Model file for the job. Use its own axes, mm. A direction names the side the tool comes from. Round coordinates to 2 decimals unless told otherwise and drop trailing zeros. Order: outer loops, then holes, each group sorted by start corner. A loop starts at its lowest first (then second) coordinate and runs counter-clockwise, first axis right, second up. Notation, with made-up numbers: (-2.75, -5) - (29.25, -5) arc R32 ccw to (29.25, 23) - close; hole circle Ø8 at (72, -37). An arc over 180 degrees is marked (long way). Answer as CSV lines item,"result". Start each with the question number.
1. Pull direction Z, two halves, no side cores. Call faces 1 (the face through (-1, 3, -63.5)), 2 (the face through (-1, 6.35, -1)), 3 (the face through (22.225, 3, -44)): released by +Z, released by -Z, zero draft, split by the parting line, or undercut.
2. 3-axis set-ups, long thin cutter, end or side, ignore diameter. For faces 4 (the face through (-36.141, 3.131, 28.333)), 5 (the face through (22.225, 3, -25)): which of +Z, -Z, +X, -X, +Y, -Y reach the whole face in a straight line?
3. Pin check, flat tips, straight feed: pin 1 Ø5 at (x, z) = (15.875, 0) entering from +Y (3 decimals); pin 2 Ø1.3 at (y, z) = (4, -7.5) entering from +X (3 decimals). Stop position of each tip, or through.
4. Wall check: line 1 along X through (y, z) = (4.5, 0) (3 decimals); line 2 along Z through (x, y) = (29, 5); line 3 along Z through (x, y) = (30, 3.5). Give the ranges that are in metal, low to high. Write a range as [from, to].
5. Band-saw the part on A-A on z = 0. List the corners of the cut face in (x, y) (3 decimals).
6. Band-saw the part on B-B on z = -26. List the corners of the cut face in (x, y) (3 decimals).
```python
from build123d import *

# Parameters (mm, degrees)
SKETCH1_W           = 95.25
SKETCH1_H           = 127
SKETCH1_R           = 3.175
BOSS_EXTRUDE1_DEPTH = 6.35
SKETCH2_R           = 2.15265
CUT_EXTRUDE1_DEPTH  = 25.4


with BuildPart() as part:
    # Sketch1 → Boss-Extrude1 (new body)
    with BuildSketch(Plane(origin=(0, 0, 0), x_dir=(1, 0, 0), z_dir=(0, 1, 0))):
        Rectangle(SKETCH1_W, SKETCH1_H)
        with Locations(Location((-34.925, 0, 0), (0, 0, 270))):
            Circle(SKETCH1_R, mode=Mode.SUBTRACT)
        with Locations(Location((-9.525, 0, 0), (0, 0, 270))):
            Circle(SKETCH1_R, mode=Mode.SUBTRACT)
        with Locations(Location((15.875, 0, 0), (0, 0, 270))):
            Circle(SKETCH1_R, mode=Mode.SUBTRACT)
        with Locations(Location((-9.525, -25.4, 0), (0, 0, 270))):
            Circle(SKETCH1_R, mode=Mode.SUBTRACT)
        with Locations(Location((15.875, -25.4, 0), (0, 0, 270))):
            Circle(SKETCH1_R, mode=Mode.SUBTRACT)
        with Locations(Location((-9.525, -50.8, 0), (0, 0, 270))):
            Circle(SKETCH1_R, mode=Mode.SUBTRACT)
        with Locations(Location((15.875, -50.8, 0), (0, 0, 270))):
            Circle(SKETCH1_R, mode=Mode.SUBTRACT)
        with Locations(Location((-34.925, -25.4, 0), (0, 0, 270))):
            Circle(SKETCH1_R, mode=Mode.SUBTRACT)
        with Locations(Location((-34.925, -50.8, 0), (0, 0, 270))):
            Circle(SKETCH1_R, mode=Mode.SUBTRACT)
    extrude(amount=BOSS_EXTRUDE1_DEPTH)

    # Sketch2 → Cut-Extrude1 (cut)
    with BuildSketch(Plane(origin=(47.625, 0, 0), x_dir=(0, 0, -1), z_dir=(1, 0, 0))):
        with Locations((44.44238, 3.175)):
            Circle(SKETCH2_R)
        with Locations((25.39238, 3.175)):
            Circle(SKETCH2_R)
        with Locations((6.34238, 3.175)):
            Circle(SKETCH2_R)
    extrude(amount=-CUT_EXTRUDE1_DEPTH, mode=Mode.SUBTRACT)


solid = part.part
```
Reply:
1,face 1,"released by -Z"
1,face 2,"zero draft"
1,face 3,"undercut"
2,face 4,"+Y, -Y"
2,face 5,"+X"
3,pin 1,"passes through"
3,pin 2,"stops at x = 22.225"
4,line 1,"x = [-47.625, -38.1], [-31.75, -12.7], [-6.35, 12.7], [19.05, 47.625]"
4,line 2,"z = [-63.5, -45.58], [-43.3, -26.53], [-24.25, -7.48], [-5.2, 63.5]"
4,line 3,"z = [-63.5, -46.57], [-42.31, -27.52], [-23.26, -8.47], [-4.21, 63.5]"
5,outline,"(-47.625, 0) - (-38.1, 0) - (-38.1, 6.35) - (-47.625, 6.35) - close; (-31.75, 0) - (-12.7, 0) - (-12.7, 6.35) - (-31.75, 6.35) - close; (-6.35, 0) - (12.7, 0) - (12.7, 6.35) - (-6.35, 6.35) - close; (19.05, 0) - (47.625, 0) - (47.625, 6.35) - (19.05, 6.35) - close"
6,outline,"(-47.625, 0) - (47.625, 0) - (47.625, 1.11) - (22.225, 1.11) - (22.225, 5.24) - (47.625, 5.24) - (47.625, 6.35) - (-47.625, 6.35) - close"
